```python
from build123d import *

# Parameters (mm, degrees)
SKETCH1_W               = 42.5
SKETCH1_H               = 3
SKETCH1_H_2             = 2
SKETCH3_R               = 37
CUT_EXTRUDE2_DEPTH      = 62
CUT_EXTRUDE3_START      = 42.5
SKETCH5_R               = 18
CUT_EXTRUDE3_DEPTH      = 10
BOSS_EXTRUDE1_START     = 25
SKETCH5_5_R             = 18
BOSS_EXTRUDE1_DEPTH     = 15
CUT_EXTRUDE4_DEPTH      = 86.76414545
CUT_EXTRUDE4_DEPTH_BACK = 86.76414545
SKETCH5_6_R             = 11


with BuildPart() as part:
    # Sketch1 → Revolve1 (revolve)
    with BuildSketch(Plane(origin=(0, 0, 0), x_dir=(0, 0, -1), z_dir=(1, 0, 0))):
        Polygon((0, -6.557009126), (0, 31.442990874), (-46.5, 31.442990874), (-46.5, -6.557009126), (-42.5, -6.557009126), align=None)
        with Locations((-21.25, 33.942990874)):
            Rectangle(SKETCH1_W, SKETCH1_H)
        with Locations((-21.25, 38.942990874)):
            Rectangle(SKETCH1_W, SKETCH1_H)
        with Locations((-21.25, 48.942990874)):
            Rectangle(SKETCH1_W, SKETCH1_H)
        with BuildLine():
            Line((0, 52.442990874), (0, 54.442990874))
            ThreePointArc((0, 54.442990874), (-23.311799933, 54.879839317), (-46.5, 52.442990874))
            Line((-46.5, 52.442990874), (0, 52.442990874))
        make_face()
        Polygon((0, 50.442990874), (0, 52.442990874), (-46.5, 52.442990874), (-46.5, 50.442990874), (-42.5, 50.442990874), align=None)
        Polygon((0, 45.442990874), (0, 47.442990874), (-42.5, 47.442990874), (-46.5, 47.442990874), (-46.5, 45.442990874), (-42.5, 45.442990874), align=None)
        with Locations((-21.25, 43.942990874)):
            Rectangle(SKETCH1_W, SKETCH1_H)
        Polygon((0, 40.442990874), (0, 42.442990874), (-42.5, 42.442990874), (-46.5, 42.442990874), (-46.5, 40.442990874), (-42.5, 40.442990874), align=None)
        Polygon((0, 35.442990874), (0, 37.442990874), (-42.5, 37.442990874), (-46.5, 37.442990874), (-46.5, 35.442990874), (-42.5, 35.442990874), align=None)
        Polygon((0, 31.442990874), (0, 32.442990874), (-42.5, 32.442990874), (-46.5, 32.442990874), (-46.5, 31.442990874), align=None)
        Polygon((0, -13.557009126), (0, -8.557009126), (-42.5, -8.557009126), (-46.5, -8.557009126), (-46.5, -13.557009126), (-42.5, -13.557009126), align=None)
        with Locations((-21.25, -7.557009126)):
            Rectangle(SKETCH1_W, SKETCH1_H_2)
    revolve(axis=Axis((0, 54.442990874, 0), (0, -1, 0)))

    # Sketch3 → Cut-Extrude2 (cut)
    with BuildSketch(Plane.XZ.offset(13.557009126)):
        with Locations(Location((0, 0, 0), (0, 0, 270))):
            Circle(SKETCH3_R)
    extrude(amount=-CUT_EXTRUDE2_DEPTH, mode=Mode.SUBTRACT)

    # Sketch5 → Cut-Extrude3 (cut)
    with BuildSketch(Plane.XY.offset(CUT_EXTRUDE3_START)):
        with Locations(Location((0, 12.942990874, 0), (0, 0, 270))):
            Circle(SKETCH5_R)
    cut_extrude3 = extrude(amount=CUT_EXTRUDE3_DEPTH, mode=Mode.SUBTRACT)

    # Mirror1: Cut-Extrude3 across plane
    add(cut_extrude3.mirror(Plane.XY), mode=Mode.SUBTRACT)

    # Sketch5_5 → Boss-Extrude1 (add)
    with BuildSketch(Plane.XY.offset(BOSS_EXTRUDE1_START)):
        with Locations(Location((0, 12.942990874, 0), (0, 0, 270))):
            Circle(SKETCH5_5_R)
    boss_extrude1 = extrude(amount=BOSS_EXTRUDE1_DEPTH)

    # Mirror2: Boss-Extrude1 across plane
    add(boss_extrude1.mirror(Plane.XY))

    # Sketch5_6 → Cut-Extrude4 (cut, two sides: drawn at the far end of the back side and taken through both)
    with BuildSketch(Plane.XY.offset(-CUT_EXTRUDE4_DEPTH_BACK)):
        with Locations((0, 12.942990874)):
            Circle(SKETCH5_6_R)
    extrude(amount=CUT_EXTRUDE4_DEPTH + CUT_EXTRUDE4_DEPTH_BACK, mode=Mode.SUBTRACT)


solid = part.part
```
Work out the finished part from the listing and answer in its coordinate system (mm). A direction names the side the tool comes from. Round coordinates to 2 decimals unless told otherwise and drop trailing zeros. Write each loop counter-clockwise with the first axis right and the second up, starting at its lowest first coordinate (ties: lowest second). Pieces come first, ordered by that corner, then holes.
1) A cutting plane is placed at D-D on y = 4. Determine the outline of the cut face in (x, z).
2) Flat-ended cylindrical pins translate along their axes: P1, Ø10, axis at x = -13.5, y = 28.5, coming from the +Z side; P2, Ø1.5, axis at x = 28, y = 44.5, coming from the +Z side; P3, Ø8, axis at x = 13, y = 18.5, coming from the -Z side. Find the tip coordinate at first contact, or state that the pin passes through.
3) A cutting plane is placed at B-B on x = 4. Give the number of separate pieces and of enclosed holes in the cut face, and give its area (3 significant figures).
4) Which of the six approach directions +Z, -Z, +X, -X, +Y, -Y give full straight-line access (tool end or side, diameter ignored) to faces 1 (the face through (-15.97, 4.64, -43.14)), 2 (the face through (-8, 21, 42.5)), 3 (the face through (25.861, 43.964, -33.727))?
5) A cutting plane is placed at A-A on y = 11. Determine the outline of the cut face in (x, z).
6) Consider probe 1 along Z at (x, y) = (11.5, 8); probe 2 along Y at (x, z) = (0, -34); probe 3 along Y at (x, z) = (-4, -31). Determine where each line is inside the solid, lowest interval first.
7) Determine the mould class of faces 4 (the face through (25.861, -7.543, -33.727)), 5 (the face through (-22.514, 17.009, 29.362)), 6 (the face through (17.847, 15.286, 29.583)), 7 (the face through (38, 42.443, -20)) for opening direction Z: pulls with the +Z half, pulls with the -Z half, needs draft (parallel to the pull), parting line crosses it, or undercut.
Entries:
1. outline: (-15.62, -43.8) - (-15.62, -42.5) - (-6.4, -42.5) - (-6.4, -25) - (-15.62, -25) - (-15.62, -33.54) arc R37 cw to (-15.62, 33.54) - (-15.62, 25) - (-6.4, 25) - (-6.4, 42.5) - (-15.62, 42.5) - (-15.62, 43.8) arc R46.5 ccw to start; (6.4, -42.5) - (15.62, -42.5) - (15.62, -43.8) arc R46.5 ccw to (15.62, 43.8) - (15.62, 42.5) - (6.4, 42.5) - (6.4, 25) - (15.62, 25) - (15.62, 33.54) arc R37 cw to (15.62, -33.54) - (15.62, -25) - (6.4, -25) - close
2. P1: stops at z = 45.71
2. P2: stops at z = 32.61
2. P3: stops at z = -43.64
3. separate pieces: 3
3. enclosed holes: 0
3. area: 1,470 mm2
4. face 1: -Z
4. face 2: +Z
4. face 3: none
5. outline: (-17.89, -42.92) - (-17.89, -42.5) - (-10.83, -42.5) - (-10.83, -25) - (-17.89, -25) - (-17.89, -32.38) arc R37 cw to (-17.89, 32.38) - (-17.89, 25) - (-10.83, 25) - (-10.83, 42.5) - (-17.89, 42.5) - (-17.89, 42.92) arc R46.5 ccw to start; (10.83, -42.5) - (17.89, -42.5) - (17.89, -42.92) arc R46.5 ccw to (17.89, 42.92) - (17.89, 42.5) - (10.83, 42.5) - (10.83, 25) - (17.89, 25) - (17.89, 32.38) arc R37 cw to (17.89, -32.38) - (17.89, -25) - (10.83, -25) - close
6. probe 1: z = -42.5 to -25, 25 to 42.5
6. probe 2: y = -5.06 to 1.94, 23.94 to 30.94, 48.44 to 54.12
6. probe 3: y = -4.61 to 2.7, 23.19 to 30.49, 48.44 to 54.37
7. face 4: parting line crosses it
7. face 5: undercut
7. face 6: undercut
7. face 7: needs draft
